Geometry: see drawing. Coordinates: mm, zero at the bounding-box minimum. A direction names the side the tool comes from. Give positions to 0.01 mm unless a question says otherwise; leave off trailing zeros. Loops run counter-clockwise (first coordinate to the right, second up) from the corner with the lowest first, then second, coordinate; pieces in that order, holes last. Notation, with made-up numbers: (-8.75, 50) -> (50.25, 50) arc R17 cw to (50.25, 70) -> close; hole circle Ø8 at (50.25, 84). An arc over 180 degrees is marked (long way). Use CSV: the item, a comma, the result in double quotes.
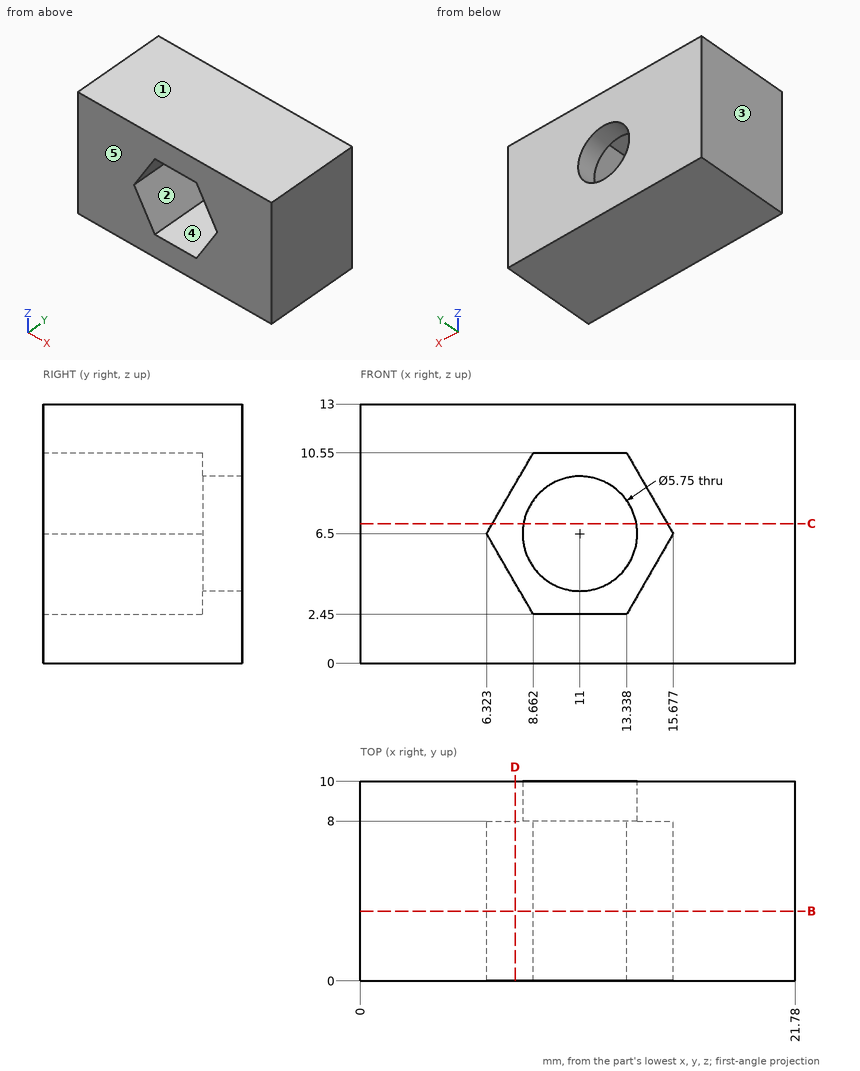
1) Contact query for flat-ended pins moving along their axis: pin 1 (1.5 mm diameter, centred on x = 8.5, z = 5, fed in from -Y); pin 2 (5 mm diameter, centred on x = 11, z = 6.5, fed in from +Y); pin 3 (5 mm diameter, centred on x = 10, y = 5.5, fed in from -Z). Output: stop coordinate, or through.
From the geometry:
pin 1,"stops at y = 8"
pin 2,"passes through"
pin 3,"stops at z = 0"
2) Section query D-D (x = 7.75). Return loops of the section in (y, z).
From the geometry:
outline,"(0, 0) -> (10, 0) -> (10, 13) -> (0, 13) -> (0, 8.97) -> (8, 8.97) -> (8, 4.03) -> (0, 4.03) -> close"
3) Section query C-C (z = 7). Return loops of the section in (x, y), then the cut area to 3 significant figures.
From the geometry:
outline,"(0, 0) -> (6.61, 0) -> (6.61, 8) -> (8.17, 8) -> (8.17, 10) -> (0, 10) -> close; (13.83, 8) -> (15.39, 8) -> (15.39, 0) -> (21.78, 0) -> (21.78, 10) -> (13.83, 10) -> close"
area,"136 mm^2"
4) Reachability of the marked faces 4 and 5 from +Z, -Z, +X, -X, +Y, -Y: full face, straight path, thin tool, end or side. Return the list, or none.
From the geometry:
face 4,"-Y"
face 5,"+Z, -Z, +X, -X, -Y"
5) Mould query, pull axis X, two halves, no side actions, for the marked faces 1, 2 and 3. Classes: pulls with the +X half, pulls with the -X half, needs draft (parallel to the pull), parting line crosses it, or undercut.
From the geometry:
face 1,"needs draft"
face 2,"undercut"
face 3,"pulls with the -X half"
6) Section query B-B (y = 3.5). Return loops of the section in (x, z), then the cut area to 3 significant figures.
From the geometry:
outline,"(0, 0) -> (21.78, 0) -> (21.78, 13) -> (0, 13) -> close; hole (6.32, 6.5) -> (8.66, 2.45) -> (13.34, 2.45) -> (15.68, 6.5) -> (13.34, 10.55) -> (8.66, 10.55) -> close"
area,"226 mm^2"
7) Ray query, line 1 (Z direction, x = 10.75, y = 0.5); line 2 (Z direction, x = 11, y = 9.3) (1 decimal); line 3 (X direction, y = 0.75, z = 3.25). Return the intervals inside material, ascending.
From the geometry:
line 1,"z = 0 to 2.45, 10.55 to 13"
line 2,"z = 0 to 3.6, 9.4 to 13"
line 3,"x = 0 to 8.2, 13.8 to 21.78"
